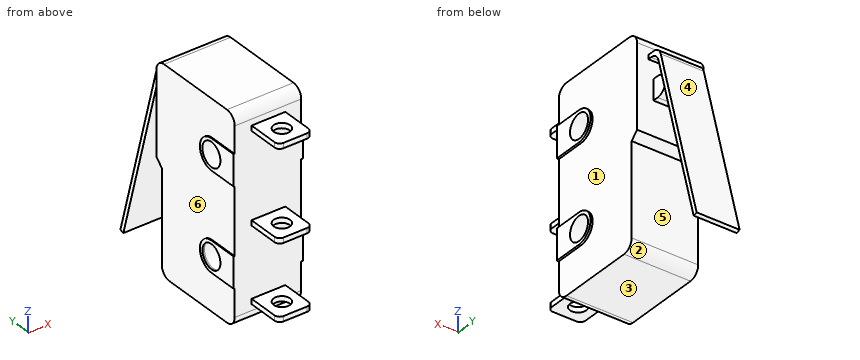
```python
from build123d import *

# Parameters (mm, degrees)
EXTRUDE_1_DEPTH      = 3.2
EXTRUDE_1_DEPTH_BACK = 3.3
SKETCH_1_W           = 19.8
SKETCH_1_H           = 10.2
CUT_EXTRUDE_1_DEPTH  = 13.894572502
FILLET_1_R           = 1
EXTRUDE_2_DEPTH      = 1.65
EXTRUDE_2_DEPTH_BACK = 1.65
SKETCH_4_W           = 0.5
SKETCH_4_H           = 3.5
FILLET_2_R           = 0.5
SKETCH_5_R           = 0.8
CUT_EXTRUDE_2_DEPTH  = 21.398284242
SKETCH_8_R           = 1.175
CUT_EXTRUDE_3_DEPTH  = 15.636256352
EXTRUDE_3_DEPTH      = 2.1
EXTRUDE_3_DEPTH_BACK = 2.1
EXTRUDE_5_DEPTH      = 1.6
EXTRUDE_5_DEPTH_BACK = 1.5
FILLET_3_R           = 1
EXTRUDE_START        = 0.2
SKETCH_9_R           = 1.175
EXTRUDE_6_DEPTH      = 0.2


with BuildPart() as part:
    # 草图1 → 凸台-拉伸1 (new, two sides: drawn at the far end of the back side and taken through both)
    with BuildSketch(Plane(origin=(0, 0, 0), x_dir=(0, 0, -1), z_dir=(1, 0, 0)).offset(-EXTRUDE_1_DEPTH_BACK)):
        Rectangle(SKETCH_1_W, SKETCH_1_H)
    extrude(amount=EXTRUDE_1_DEPTH + EXTRUDE_1_DEPTH_BACK)

    # 草图2 → 切除-拉伸1 (cut, through all)
    with BuildSketch(Plane(origin=(3.2, 0, 0), x_dir=(0, 0, -1), z_dir=(1, 0, 0))):
        Polygon((-0.8, 5.1), (-0.1, 4.4), (9.9, 4.4), (9.9, 5.1), align=None)
    extrude(amount=-CUT_EXTRUDE_1_DEPTH, mode=Mode.SUBTRACT)

    # 圆角1
    fillet_1_edges = [part.edges().sort_by_distance(p)[0] for p in [
        (-0.05, 4.4, -9.9),
        (-0.05, -5.1, -9.9),
        (-0.05, -5.1, 9.9),
        (-0.05, 5.1, 9.9),
    ]]
    fillet(fillet_1_edges, radius=FILLET_1_R)

    # 草图4 → 凸台-拉伸2 (add, two sides: drawn at the far end of the back side and taken through both)
    with BuildSketch(Plane(origin=(0, 0, 0), x_dir=(0, 0, -1), z_dir=(1, 0, 0)).offset(-EXTRUDE_2_DEPTH_BACK)):
        with Locations((-8.05, -6.85)):
            Rectangle(SKETCH_4_W, SKETCH_4_H)
        with Locations((0.75, -6.85)):
            Rectangle(SKETCH_4_W, SKETCH_4_H)
        with Locations((8.05, -6.85)):
            Rectangle(SKETCH_4_W, SKETCH_4_H)
    extrude(amount=EXTRUDE_2_DEPTH + EXTRUDE_2_DEPTH_BACK)

    # 圆角2
    fillet_2_edges = [part.edges().sort_by_distance(p)[0] for p in [
        (-1.65, -8.6, 8.05),
        (1.65, -8.6, 8.05),
        (-1.65, -8.6, -0.75),
        (1.65, -8.6, -0.75),
        (1.65, -8.6, -8.05),
        (-1.65, -8.6, -8.05),
    ]]
    fillet(fillet_2_edges, radius=FILLET_2_R)

    # 草图5 → 切除-拉伸2 (cut, through all)
    with BuildSketch(Plane.XY.offset(8.3)):
        with Locations(Location((0, -6.85, 0), (0, 0, 270))):
            Circle(SKETCH_5_R)
    extrude(amount=-CUT_EXTRUDE_2_DEPTH, mode=Mode.SUBTRACT)

    # 草图8 → 切除-拉伸3 (cut, through all)
    with BuildSketch(Plane(origin=(3.2, 0, 0), x_dir=(0, 0, -1), z_dir=(1, 0, 0))):
        with Locations((-4.8, -2.2)):
            Circle(SKETCH_8_R)
        with Locations((4.7, -2.2)):
            Circle(SKETCH_8_R)
    extrude(amount=-CUT_EXTRUDE_3_DEPTH, mode=Mode.SUBTRACT)

    # 草图6 → 凸台-拉伸3 (add, two sides: drawn at the far end of the back side and taken through both)
    with BuildSketch(Plane(origin=(0, 0, 0), x_dir=(0, 0, -1), z_dir=(1, 0, 0)).offset(-EXTRUDE_3_DEPTH_BACK)):
        Polygon((-7.775241221, 6.217237719), (9.805291462, 11.014106611), (9.7, 11.4), (-8.175241221, 6.52271954), (-8.175241221, 5.1), (-7.775241221, 5.1), align=None)
    extrude(amount=EXTRUDE_3_DEPTH + EXTRUDE_3_DEPTH_BACK)

    # 草图7 → 凸台-拉伸5 (add, two sides: drawn at the far end of the back side and taken through both)
    with BuildSketch(Plane(origin=(0, 0, 0), x_dir=(0, 0, -1), z_dir=(1, 0, 0)).offset(-EXTRUDE_5_DEPTH_BACK)):
        with BuildLine():
            Line((-4.126745085, 5.653223192), (-4.126745085, 5.1))
            Line((-4.126745085, 5.1), (-6.126745085, 5.1))
            Line((-6.126745085, 5.1), (-6.126745085, 5.653223192))
            ThreePointArc((-6.126745085, 5.653223192), (-5.126745085, 6.653223192), (-4.126745085, 5.653223192))
        make_face()
    extrude(amount=EXTRUDE_5_DEPTH + EXTRUDE_5_DEPTH_BACK)

    # 圆角3
    fillet_3_edges = [part.edges().sort_by_distance(p)[0] for p in [
        (0, 6.217237719, 7.775241221),
        (0, 6.52271954, 8.175241221),
    ]]
    fillet(fillet_3_edges, radius=FILLET_3_R)

    # 草图9 → 凸台-拉伸6 (add)
    # profile 1 of 2: a face of its own
    with BuildSketch(Plane(origin=(3.2, 0, 0), x_dir=(0, 0, -1), z_dir=(1, 0, 0)).offset(EXTRUDE_START)):
        with BuildLine():
            Line((-3.3, -2.2), (-3.3, -5.1))
            Line((-3.3, -5.1), (-6.3, -5.1))
            Line((-6.3, -5.1), (-6.3, -2.2))
            ThreePointArc((-6.3, -2.2), (-4.8, -0.7), (-3.3, -2.2))
        make_face()
        with Locations((-4.8, -2.2)):
            Circle(SKETCH_9_R, mode=Mode.SUBTRACT)
    # profile 2 of 2: a face of its own
    with BuildSketch(Plane(origin=(3.2, 0, 0), x_dir=(0, 0, -1), z_dir=(1, 0, 0)).offset(EXTRUDE_START)):
        with BuildLine():
            Line((3.2, -2.2), (3.2, -5.1))
            Line((3.2, -5.1), (6.2, -5.1))
            Line((6.2, -5.1), (6.2, -2.2))
            ThreePointArc((6.2, -2.2), (4.7, -0.7), (3.2, -2.2))
        make_face()
        with Locations((4.7, -2.2)):
            Circle(SKETCH_9_R, mode=Mode.SUBTRACT)
    extrude_6 = extrude(amount=-EXTRUDE_6_DEPTH)

    # 镜向1: 凸台-拉伸6 across plane
    add(extrude_6.mirror(Plane(origin=(0, 0, 0), x_dir=(0, 0, 1), z_dir=(1, 0, 0))))


solid = part.part
```
Source: CAD feature listing. Evaluate the final solid. Frame: model axes, mm. Face numbers are marked on the shaded views. A direction names the side the tool comes from. Give positions to 0.01 mm unless a question says otherwise; leave off trailing zeros. Loops run counter-clockwise (first coordinate to the right, second up) from the corner with the lowest first, then second, coordinate; pieces in that order, holes last. Notation, with made-up numbers: (-23.75, 53) - (-4.75, 53) arc R4 ccw to (-4.75, 58) - close; hole circle Ø10 at (83, 31.25). An arc over 180 degrees is marked (long way). Use CSV: the item, a comma, the result in double quotes.
1) Pin query (flat end, axial travel): P1, Ø1.8, axis at x = 0, y = -6.85, coming from the +Z side; P2, Ø1.5, axis at y = 7, z = -1.5, coming from the -X side; P3, Ø4, axis at x = 2, z = 5, coming from the +Y side; P4, Ø4, axis at y = 2, z = 8, coming from the -X side. Return the tip coordinate at first contact, or that it passes through.
Worked out:
P1,"stops at z = 8.3"
P2,"passes through"
P3,"stops at y = 7.93"
P4,"stops at x = -3.3"
2) Line query: line 1 (Y direction, x = 0, z = -5.5); line 2 (Y direction, x = 0.75, z = -3.75); line 3 (Z direction, x = -0.5, y = -2.5). Output: solid intervals per line, ascending.
Worked out:
line 1,"y = -5.1 to -3.06, -1.34 to 4.4, 9.84 to 10.25"
line 2,"y = -5.1 to -2.89, -1.51 to 4.4, 9.36 to 9.78"
line 3,"z = -9.9 to -5.84, -3.56 to 3.66, 5.94 to 9.9"
3) Cut plane B-B (y = -6.85). Output: boundary loops of the cut face in (x, z).
Worked out:
outline,"(-1.65, -8.3) - (-0.8, -8.3) - (-0.8, -7.8) - (-1.65, -7.8) - close; (-1.65, -1) - (-0.8, -1) - (-0.8, -0.5) - (-1.65, -0.5) - close; (-1.65, 7.8) - (-0.8, 7.8) - (-0.8, 8.3) - (-1.65, 8.3) - close; (0.8, -8.3) - (1.65, -8.3) - (1.65, -7.8) - (0.8, -7.8) - close; (0.8, -1) - (1.65, -1) - (1.65, -0.5) - (0.8, -0.5) - close; (0.8, 7.8) - (1.65, 7.8) - (1.65, 8.3) - (0.8, 8.3) - close"
4) Set-up query: the marked faces 1, 2 and 3. Return all of +Z, -Z, +X, -X, +Y, -Y with unobstructed straight access to the full face (end or side cutting, diameter ignored); none if empty.
Worked out:
face 1,"+X, +Y"
face 2,"-Z, +X, -X"
face 3,"-Z, +X, -X, +Y, -Y"
5) Cut plane C-C (z = -2.25). Output: boundary loops of the cut face in (x, y).
Worked out:
outline,"(-3.3, -5.1) - (3.2, -5.1) - (3.2, 4.4) - (-3.3, 4.4) - close; (-2.1, 8.95) - (2.1, 8.95) - (2.1, 9.37) - (-2.1, 9.37) - close"
6) Cut plane A-A (x = 0). Count the separate pieces of the cut face and the enclosed holes in it, and give its area (3 significant figures).
Worked out:
separate pieces,"4"
enclosed holes,"2"
area,"199 mm^2"
7) Mould query, pull axis Z, two halves, no side actions, for the marked faces 4, 5 and 6. Classes: +Z half, -Z half, draft (parallel to the pull), parting line (faces both ways), or undercut.
Worked out:
face 4,"+Z half"
face 5,"draft"
face 6,"undercut"
8) Cut plane D-D (x = 2.75). Output: boundary loops of the cut face in (y, z) (3 decimals), and give its area (3 significant figures).
Worked out:
outline,"(-5.1, -8.9) arc R1 ccw to (-4.1, -9.9) - (3.4, -9.9) arc R1 ccw to (4.4, -8.9) - (4.4, 0.1) - (5.1, 0.8) - (5.1, 8.9) arc R1 ccw to (4.1, 9.9) - (-4.1, 9.9) arc R1 ccw to (-5.1, 8.9) - close; hole circle Ø2.35 at (-2.2, -4.7); hole circle Ø2.35 at (-2.2, 4.8)"
area,"185 mm^2"
